Autodesk Inventor part; units mm, degrees
ref_plane "YZ Plane" through (0, 0, 0) normal (1, 0, 0) x (0, 1, 0)
ref_plane "XZ Plane" through (0, 0, 0) normal (0, 1, 0) x (-1, 0, 0)
ref_plane "XY Plane" through (0, 0, 0) normal (0, 0, 1) x (1, 0, 0)
sketch "Sketch1" plane through (0, 0, 0) normal (0, 1, 0) x (-1, 0, 0)
  line L0 (-35.56, 55) -> (35.56, 55)
  line L1 (41.91, 48.65) -> (41.91, -16.9)
  line L2 (3.81, -55) -> (-3.81, -55)
  line L3 (-41.91, -16.9) -> (-41.91, 48.65)
  line L4 (-41.91, 55) -> (41.91, -55) construction
  line L5 (41.91, 55) -> (-41.91, -55) construction
  arc A0 (3.81, -55) -> (41.91, -16.9) centre (3.81, -16.9) ccw
  arc A1 (-41.91, -16.9) -> (-3.81, -55) centre (-3.81, -16.9) ccw
  arc A2 (41.91, 48.65) -> (35.56, 55) centre (35.56, 48.65) ccw
  arc A3 (-35.56, 55) -> (-41.91, 48.65) centre (-35.56, 48.65) ccw
  line L6 (113.65, -53.500747) -> (-33.65, 85.250747) construction
  line L7 (-33.65, -53.500747) -> (113.65, 85.250747) construction
  line L8 (52.07, -9.508324) -> (31.75, -9.508324)
  line L9 (31.75, -9.508324) -> (31.75, 20.971676)
  line L10 (31.75, 20.971676) -> (52.07, 20.971676)
  line L11 (52.07, 20.971676) -> (52.07, -9.508324)
  line L12 (52.07, -9.508324) -> (31.75, 20.971676) construction
  line L13 (31.75, -9.508324) -> (52.07, 20.971676) construction
  line L14 (0, -55) -> (0, 55)
  line L15 (33.65, -53.500747) -> (-113.65, 85.250747) construction
  line L16 (-52.07, -9.508324) -> (-31.75, -9.508324)
  line L17 (-31.75, -9.508324) -> (-31.75, 20.971676)
  line L18 (-31.75, 20.971676) -> (-52.07, 20.971676)
  line L19 (-52.07, 20.971676) -> (-52.07, -9.508324)
  line L20 (-52.07, -9.508324) -> (-31.75, 20.971676) construction
  line L21 (-31.75, -9.508324) -> (-52.07, 20.971676) construction
  line L22 (-52.07, 20.971676) -> (-31.75, 20.971676)
  line L23 (-31.75, 20.971676) -> (-31.75, -9.508324)
  line L24 (-31.75, -9.508324) -> (-52.07, -9.508324)
  line L25 (-52.07, -9.508324) -> (-52.07, 20.971676)
  line L26 (-52.07, 20.971676) -> (-31.75, -9.508324) construction
  line L27 (-31.75, 20.971676) -> (-52.07, -9.508324) construction
  point P0 (0, 0)
  point P1 (-35.56, 48.65)
  point P2 (41.91, 5.731676)
  point P3 (-41.91, 5.731676)
  point P4 (-41.91, 5.731676)
  point P5 (41.91, -9.508324)
  point P6 (41.91, 20.971676)
  point P7 (-41.91, 20.971676)
  point P8 (-41.91, -9.508324)
  dimension "d0" = 83.82
  dimension "d1" = 110
  dimension "d2" = 38.1
  dimension "d3" = 38.1
  dimension "d4" = 6.35
  dimension "d5" = 6.35
  dimension "d11" = 20.32
  dimension "d12" = 30.48
extrude "Extrusion1" add sketch "Sketch1" along normal blind 5.08 contours L0 L14 L2 A1 L3 L16 L17 L18 A3 | L0 A2 L1 L10 L9 L8 A0 L2 L14
sketch "Sketch2" plane through (0, 0, 0) normal (0, -1, 0) x (1, 0, 0)
  line L0 (-35.56, 55) -> (35.56, 55)
  line L1 (0, 55) -> (0, 47.38)
  line L2 (0, 47.38) -> (0, 31.886)
  circle A0 centre (0, 39.633) radius 7.747
  line L3 (7.747, 39.633) -> (9.017, 39.633)
  circle A1 centre (9.017, 39.633) radius 1.27
  line L4 (9.756904, 38.600798) -> (7.196844, 36.765693) construction
  spline S0 degree 1 poles (9.756904, 38.600798) (7.196844, 36.765693) knots 1 1 2 2
  line L5 (9.770215, 40.65553) -> (7.167589, 42.572673) construction
  spline S1 degree 1 poles (9.770215, 40.65553) (7.167589, 42.572673) knots 1 1 2 2
  line L6 (-7.747, 39.633) -> (-9.017, 39.633)
  circle A2 centre (-9.017, 39.633) radius 1.27
  line L7 (-9.756904, 38.600798) -> (-7.196844, 36.765693) construction
  spline S2 degree 1 poles (-9.756904, 38.600798) (-7.196844, 36.765693) knots 1 1 2 2
  line L8 (-9.770215, 40.65553) -> (-7.167589, 42.572673) construction
  spline S3 degree 1 poles (-9.770215, 40.65553) (-7.167589, 42.572673) knots 1 1 2 2
  circle A3 centre (-9.017, 39.633) radius 1.27
  line L9 (-9.770215, 40.65553) -> (-7.167589, 42.572673) construction
  spline S4 degree 1 poles (-9.770215, 40.65553) (-7.167589, 42.572673) knots 1 1 2 2
  line L10 (-9.756904, 38.600798) -> (-7.196844, 36.765693) construction
  spline S5 degree 1 poles (-9.756904, 38.600798) (-7.196844, 36.765693) knots 1 1 2 2
  line L11 (10.287, 39.633) -> (10.287, 32.454774)
  line L12 (-10.287, 39.633) -> (-10.287, 31.176127)
  circle A4 centre (7.747, 39.633) radius 1.016
  line L13 (-7.747, 39.633) -> (-9.017, 39.633)
  circle A5 centre (-9.017, 39.633) radius 1.27
  circle A6 centre (-7.747, 39.633) radius 1.016
  circle A7 centre (-7.747, 39.633) radius 1.016
  point P0 (0, 0)
  dimension "d16" = 7.62
  dimension "d17" = 15.494
  dimension "d19" = 1.27
  dimension "d27" = 2.032
  dimension "d28" = 20.574
extrude "Extrusion2" cut sketch "Sketch2" against normal blind 5.08 contours A0 A4 L2 | L2 A0 A6 | A0 A4 | A6 A0
sketch "Sketch7" plane through (0, 0, 0) normal (0, -1, 0) x (1, 0, 0)
  circle A0 centre (0, 39.633) radius 7.747
  line L0 (7.747, 39.633) -> (8.89, 39.633)
  circle A1 centre (8.89, 39.633) radius 1.143
  circle A2 centre (7.747, 39.633) radius 0.9525
  line L1 (9.653215, 40.483854) -> (7.169913, 42.566999) construction
  spline S0 degree 1 poles (9.653215, 40.483854) (7.169913, 42.566999) knots 1 1 2 2
  line L2 (9.653215, 38.782146) -> (7.169913, 36.699001) construction
  spline S1 degree 1 poles (9.653215, 38.782146) (7.169913, 36.699001) knots 1 1 2 2
  line L3 (0, 47.38) -> (0, 31.886)
  circle A3 centre (-8.89, 39.633) radius 1.143
  line L4 (-9.653215, 40.483854) -> (-7.169913, 42.566999) construction
  spline S2 degree 1 poles (-9.653215, 40.483854) (-7.169913, 42.566999) knots 1 1 2 2
  line L5 (-9.653215, 38.782146) -> (-7.169913, 36.699001) construction
  spline S3 degree 1 poles (-9.653215, 38.782146) (-7.169913, 36.699001) knots 1 1 2 2
  circle A4 centre (-8.89, 39.633) radius 1.143
  line L6 (-9.653215, 40.483854) -> (-7.169913, 42.566999) construction
  spline S4 degree 1 poles (-9.653215, 40.483854) (-7.169913, 42.566999) knots 1 1 2 2
  line L7 (-9.653215, 38.782146) -> (-7.169913, 36.699001) construction
  spline S5 degree 1 poles (-9.653215, 38.782146) (-7.169913, 36.699001) knots 1 1 2 2
  point P0 (0, 0)
  dimension "d40" = 1.143
  dimension "d41" = 1.905
sketch "Sketch7 outline for Extrusion4" plane through (0, 0, 0) normal (0, -1, 0) x (1, 0, 0)
  spline S0 degree 1 poles (-9.653215, 40.483854) (-7.169913, 42.566999) knots 0 0 1 1
  arc A0 (-7.169913, 36.699001) -> (-7.169913, 42.566999) centre (0, 39.633) cw
  spline S1 degree 1 poles (-9.653215, 38.782146) (-7.169913, 36.699001) knots 0 0 1 1
  arc A1 (-9.653215, 40.483854) -> (-9.653215, 38.782146) centre (-8.89, 39.633) ccw
  spline S2 degree 1 poles (9.653215, 40.483854) (7.169913, 42.566999) knots 0 0 1 1
  arc A2 (9.653215, 38.782146) -> (9.653215, 40.483854) centre (8.89, 39.633) ccw
  spline S3 degree 1 poles (9.653215, 38.782146) (7.169913, 36.699001) knots 0 0 1 1
  arc A3 (7.169913, 42.566999) -> (7.169913, 36.699001) centre (0, 39.633) cw
extrude "Extrusion4" cut sketch "Sketch7 outline for Extrusion4" against normal blind 2.032
sketch "Sketch8" plane through (0, 0, 0) normal (0, -1, 0) x (1, 0, 0)
  arc A0 (7.169913, 36.699001) -> (7.169913, 42.566999) centre (0, 39.633) ccw
  circle A1 centre (7.747, 39.633) radius 0.9525
  line L0 (0, 47.38) -> (0, 31.886)
  circle A2 centre (-7.747, 39.633) radius 0.9525
  circle A3 centre (-7.747, 39.633) radius 0.9525
  point P0 (0, 0)
  dimension "d44" = 1.905
extrude "Extrusion5" cut sketch "Sketch8" against normal blind 5.08
sketch "Sketch9" plane through (0, 0, 0) normal (0, -1, 0) x (1, 0, 0)
  line L0 (31.75, 20.971676) -> (31.75, -9.508324)
  line L1 (31.75, 5.731676) -> (10.338001, 5.731676)
  line L2 (0, 23.8125) -> (0, -11.1125)
  line L3 (15.875, 5.731676) -> (15.875, 18.558676)
  line L4 (41.91, 18.558676) -> (15.875, 18.558676)
  line L5 (41.91, 48.65) -> (41.91, 20.971676)
  circle A0 centre (15.875, 18.558676) radius 1.651
  circle A1 centre (15.875, -7.095324) radius 1.651
  circle A2 centre (-15.875, 18.558676) radius 1.651
  circle A3 centre (-15.875, -7.095324) radius 1.651
  point P0 (0, 0)
  dimension "d51" = 12.827
  dimension "d52" = 26.035
  dimension "d53" = 3.302
extrude "Extrusion6" cut sketch "Sketch9" against normal blind 5.08 contours A0 L3 L4 | L4 L3 A0 | A1 | A2 | A3
properties part number "micromouse"
Input: part model. Units: mm. Frame: model coordinates. A direction names the side the tool comes from. Coordinates: 2 decimals unless noted, no trailing zeros. Loops run counter-clockwise (first coordinate to the right, second up) from the corner with the lowest first, then second, coordinate; pieces in that order, holes last. Notation, with made-up numbers: (9, -21.75) -> (38, -21.75) arc R20 ccw to (38, 15.25) -> close; hole circle Ø3 at (22, -14). An arc over 180 degrees is marked (long way). One line per item, written item: value.
(1) Ray query, line 1 along X through (y, z) = (1.65, 18); line 2 along X through (y, z) = (4.8, 17.5); line 3 along Z through (x, y) = (-33, 2.5). Return the intervals inside material, ascending.
Answer below:
line 1: x = -31.75 to -17.43, -14.32 to 14.32, 17.43 to 31.75
line 2: x = -31.75 to -17.14, -14.61 to 14.61, 17.14 to 31.75
line 3: z = -41.39 to -9.51, 20.97 to 55
(2) Set-up query: faces 1 (the face through (-37, 3, -9.508)), 2 (the face through (31.75, 3, 6)), 3 (the face through (-0.157, 2.504, 31.888)). Return all of +Z, -Z, +X, -X, +Y, -Y with unobstructed straight access to the full face (end or side cutting, diameter ignored); none if empty.
Answer below:
face 1: -X, +Y, -Y
face 2: +X, +Y, -Y
face 3: +Y, -Y
(3) Cut plane B-B (x = -33.5). Output: boundary loops of the cut face in (y, z), then the cut area to 3 significant figures.
Answer below:
outline: (0, -40.78) -> (5.08, -40.78) -> (5.08, -9.51) -> (0, -9.51) -> close; (0, 20.97) -> (5.08, 20.97) -> (5.08, 55) -> (0, 55) -> close
area: 332 mm2
(4) Cut plane C-C (z = -4). Output: boundary loops of the cut face in (x, y), then the cut area to 3 significant figures.
Answer below:
outline: (-31.75, 0) -> (31.75, 0) -> (31.75, 5.08) -> (-31.75, 5.08) -> close
area: 323 mm2
(5) Cut plane D-D (x = 29). Output: boundary loops of the cut face in (y, z).
Answer below:
outline: (0, -45.48) -> (5.08, -45.48) -> (5.08, 55) -> (0, 55) -> close
(6) Pin query (flat end, axial travel): pin 1 Ø1.5 at (y, z) = (2, 11) entering from -X; pin 2 Ø2.5 at (x, y) = (-35, 3.5) entering from -Z; pin 3 Ø2.5 at (x, y) = (37.5, 2.5) entering from -Z. Return the tip coordinate at first contact, or that it passes through.
Answer below:
pin 1: stops at x = -31.75
pin 2: stops at z = -40.46
pin 3: stops at z = -36.88
(7) Cut plane A-A (y = 3.55). Give the number of separate pieces and of enclosed holes in the cut face, then the cut area to 3 significant figures.
Answer below:
separate pieces: 1
enclosed holes: 5
area: 7,730 mm2
(8) Draft query along Z for faces 4 (the face through (-9, 2.032, 40)), 5 (the face through (30.45, 2.5, -44.14)), 6 (the face through (-31.75, 3, 6)), 7 (the face through (1, 0, 1)). Return one class per face: pulls with the +Z half, pulls with the -Z half, needs draft (parallel to the pull), parting line crosses it, or undercut.
Answer below:
face 4: undercut
face 5: pulls with the -Z half
face 6: undercut
face 7: needs draft
